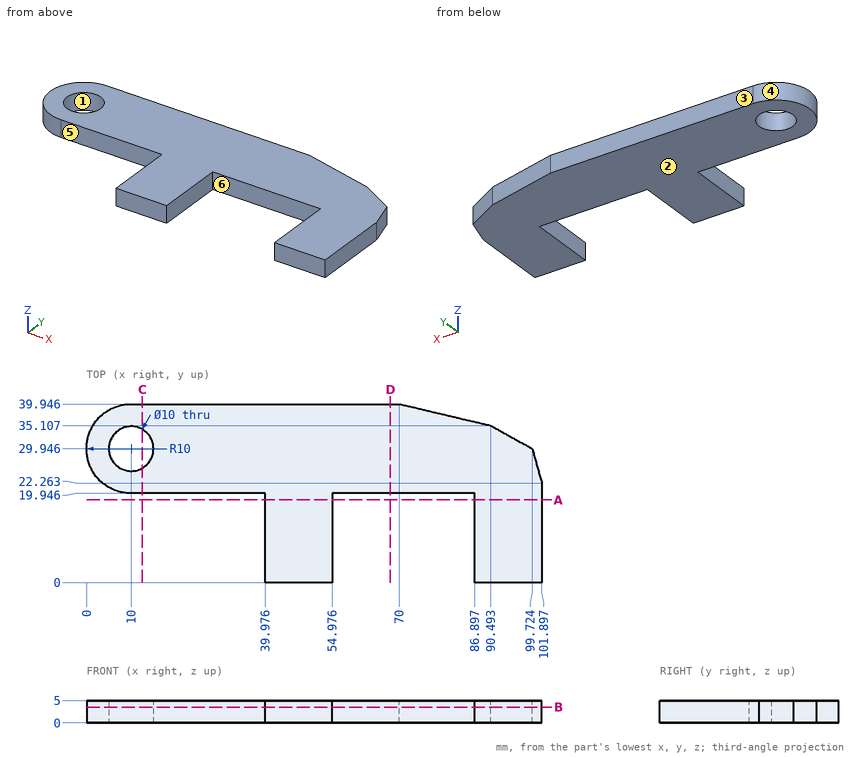
Part print with two shaded views. Sizes in mm from the minimum x, y, z corner. A direction names the side the tool comes from. Coordinates: 2 decimals unless noted, no trailing zeros. Loops run counter-clockwise (first coordinate to the right, second up) from the corner with the lowest first, then second, coordinate; pieces in that order, holes last. Notation, with made-up numbers: (-5, 5.25) -> (3, 5.25) arc R15 cw to (3, 19.25) -> close; hole circle Ø10 at (-24, 11). An arc over 180 degrees is marked (long way). Answer as a JSON object with one key per item and string values.
Q1. Pull direction Y, two halves, no side cores. Call the marked faces 1, 2 and 3: released by +Y, released by -Y, zero draft, split by the parting line, or undercut.
Report:
{"face 1": "undercut", "face 2": "zero draft", "face 3": "released by +Y"}
Q2. Cut at C-C (x = 12.5). List the corners of the cut face in (y, z).
Report:
{"outline": "(19.95, 0) -> (25.62, 0) -> (25.62, 5) -> (19.95, 5) -> close; (34.28, 0) -> (39.95, 0) -> (39.95, 5) -> (34.28, 5) -> close"}
Q3. Cut at D-D (x = 68). List the corners of the cut face in (y, z), and give its area (3 significant figures).
Report:
{"outline": "(19.95, 0) -> (39.95, 0) -> (39.95, 5) -> (19.95, 5) -> close", "area": "100 mm2"}
Q4. 3-axis set-ups, long thin cutter, end or side, ignore diameter. For the marked faces 4, 5 and 6: which of +Z, -Z, +X, -X, +Y, -Y reach the whole face in a straight line?
Report:
{"face 4": "+Z, -Z, -X", "face 5": "+Z, -Z, -X, -Y", "face 6": "+Z, -Z, -Y"}
Q5. Cut at A-A (y = 18.5). List the corners of the cut face in (x, z).
Report:
{"outline": "(39.98, 0) -> (54.98, 0) -> (54.98, 5) -> (39.98, 5) -> close; (86.9, 0) -> (101.9, 0) -> (101.9, 5) -> (86.9, 5) -> close"}
Q6. Flat gauge pins, fed straight in: P1, Ø6, axis at x = 10, y = 29.95, coming from the +Z side; P2, Ø2.5, axis at y = 7.5, z = 3, coming from the -X side; P3, Ø1.5, axis at y = 25.5, z = 4.5, coming from the +X side. Where does each tip first touch, or does it go through?
Report:
{"P1": "passes through", "P2": "stops at x = 39.98", "P3": "stops at x = 101.19"}
Q7. Probe probe 1 along X at (y, z) = (5.5, 3.75); probe 2 along Y at (x, z) = (10, 4.05); probe 3 along X at (y, z) = (29.5, 0.75). List the from-to ranges inside material, lowest first.
Report:
{"probe 1": "x = 39.98 to 54.98, 86.9 to 101.9", "probe 2": "y = 19.95 to 24.95, 34.95 to 39.95", "probe 3": "x = 0.01 to 5.02, 14.98 to 99.85"}
Q8. Cut at B-B (z = 3.5). List the corners of the cut face in (x, y), and give its area (3 significant figures).
Report:
{"outline": "(10, 19.95) -> (39.98, 19.95) -> (39.98, 0) -> (54.98, 0) -> (54.98, 19.95) -> (86.9, 19.95) -> (86.9, 0) -> (101.9, 0) -> (101.9, 22.26) -> (99.72, 29.95) -> (90.49, 35.11) -> (70, 39.95) -> (10, 39.95) arc R10 ccw to start; hole circle Ø10 at (10, 29.95)", "area": "2,370 mm2"}
